Work out the finished part from the listing and answer in its coordinate system (mm). Face numbers are marked on the shaded views. Round coordinates to 2 decimals unless told otherwise and drop trailing zeros. Order: outer loops, then holes, each group sorted by start corner. A loop starts at its lowest first (then second) coordinate and runs counter-clockwise, first axis right, second up. Notation, with made-up numbers: M 72,35.5 L 113,35.5 A13 ccw 113,50.5 Z; hole C 0.25,19 d10. An arc over 180 degrees is marked long. Answer as a JSON object with one key per item and string values. Group by question number.
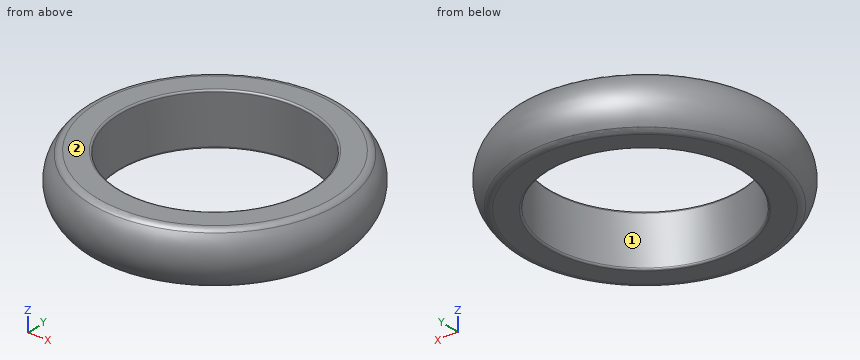
from build123d import *


with BuildPart() as f1:
    # F0 (on Front) → F1 (revolve)
    with BuildSketch(Plane.XZ):
        with BuildLine():
            ThreePointArc((-0.2, 0), (-0.058579, 0.058579), (0, 0.2))
            Line((0, 0.2), (0, 5.8))
            ThreePointArc((0, 5.8), (-0.058579, 5.941421), (-0.2, 6))
            Line((-0.2, 6), (-2.590317, 6))
            ThreePointArc((-2.590317, 6), (-2.998565, 5.912871), (-3.335673, 5.666667))
            ThreePointArc((-3.335673, 5.666667), (-4.354249, 3), (-3.335673, 0.333333))
            ThreePointArc((-3.335673, 0.333333), (-2.998565, 0.087129), (-2.590317, 0))
            Line((-2.590317, 0), (-0.2, 0))
        make_face()
    revolve(axis=Axis((11, 0, 3), (0, 0, 1)))


solid = f1.part
Item 1: Find section A-A (x = 11). Give the vertices of the cut face in (y, z), and give its area (3 significant figures).
Item 2: Consider L1, parallel to Y at x = 11, z = 4.9; L2, parallel to X at y = -10, z = 2; L3, parallel to X at y = 0, z = 3.4. Determine where each line is inside the solid, lowest interval first.
Item 3: The mould has two halves that part along X. Classify the marked faces 1 and 2: +X half, -X half, draft (parallel to the pull), parting line (faces both ways), or undercut.
Item 4: Find section D-D (z = 2.1). Give the vertices of the cut face in (x, y), and give its area (3 significant figures).
Item 5: Find section C-C (z = 4.7). Give the vertices of the cut face in (x, y).
Item 6: Find section B-B (y = 0). Give the vertices of the cut face in (x, z), and give its area (3 significant figures).
Item 7: Each of these flat-tipped pins is pushed along its axis until it touches: pin 1 (1 mm diameter, centred on x = 5.5, z = 4.5, fed in from +Y); pin 2 (2 mm diameter, centred on y = 3.5, z = 2.5, fed in from -X); pin 3 (1 mm diameter, centred on x = 18, z = 5, fed in from -Y). Where does it stop, or does it pass through?
Responses:
{
 "1": {"outline": "M -14.34,0.33 A1 ccw -13.59,0 L -11.2,0 A0.2 ccw -11,0.2 L -11,5.8 A0.2 ccw -11.2,6 L -13.59,6 A1 ccw -14.34,5.67 A4 ccw Z; M 11,0.2 A0.2 ccw 11.2,0 L 13.59,0 A1 ccw 14.34,0.33 A4 ccw 14.34,5.67 A1 ccw 13.59,6 L 11.2,6 A0.2 ccw 11,5.8 Z", "area": "47.1 mm^2"},
 "2": {"L1": "y = -14.87 to -11, 11 to 14.87", "L2": "x = -0.48 to 6.42, 15.58 to 22.48", "L3": "x = -4.33 to 0, 22 to 26.33"},
 "3": {"face 1": "undercut", "face 2": "draft"},
 "4": {"outline": "C 11,0 d30.5; hole C 11,0 d22", "area": "351 mm^2"},
 "5": {"outline": "C 11,0 d29.95; hole C 11,0 d22"},
 "6": {"outline": "M -3.34,0.33 A1 ccw -2.59,0 L -0.2,0 A0.2 ccw 0,0.2 L 0,5.8 A0.2 ccw -0.2,6 L -2.59,6 A1 ccw -3.34,5.67 A4 ccw Z; M 22,0.2 A0.2 ccw 22.2,0 L 24.59,0 A1 ccw 25.34,0.33 A4 ccw 25.34,5.67 A1 ccw 24.59,6 L 22.2,6 A0.2 ccw 22,5.8 Z", "area": "47.1 mm^2"},
 "7": {"pin 1": "stops at y = 14.29", "pin 2": "stops at x = -4.14", "pin 3": "stops at y = -13.45"}
}
